Check sheet for the modelled part. Datum: model origin and axes. Units: mm. Give positions to 0.01 mm unless a question says otherwise; leave off trailing zeros. Order: outer loops, then holes, each group sorted by start corner. A loop starts at its lowest first (then second) coordinate and runs counter-clockwise, first axis right, second up. Notation, with made-up numbers: (63.25, 25.25) - (85.25, 25.25) arc R7 ccw to (85.25, 33.25) - close; hole circle Ø1 at (18.5, -26.75). An arc over 180 degrees is marked (long way). Answer in a Markdown table with one row per item.
from build123d import *

# Parameters (mm, degrees)
F1_DEPTH = 13.2


with BuildPart() as f1:
    # F0 (on Right) → F1 (new body)
    with BuildSketch(Plane.YZ):
        with BuildLine():
            ThreePointArc((63.824689, 3.356788), (64.089665, -3.514345), (70, 0))
            ThreePointArc((70, 0), (69.14794, 2.467888), (66.954764, 3.884382))
            ThreePointArc((66.954764, 3.884382), (66.679281, 3.932074), (66.403765, 3.97957))
            ThreePointArc((66.403765, 3.97957), (65.061087, 3.888244), (63.824689, 3.356788))
        make_face()
        with BuildLine():
            ThreePointArc((69, 0), (63.87868, -2.12132), (66, 3))
            ThreePointArc((66, 3), (68.12132, 2.12132), (69, 0))
        make_face(mode=Mode.SUBTRACT)
        with BuildLine():
            ThreePointArc((66.403765, 3.97957), (66.679281, 3.932074), (66.954764, 3.884382))
            ThreePointArc((66.954764, 3.884382), (66.68093, 3.941616), (66.403765, 3.97957))
        make_face()
        with BuildLine():
            ThreePointArc((-64.71288, 2.709856), (-0.470808, 8.340736), (63.824689, 3.356788))
            ThreePointArc((63.824689, 3.356788), (65.061087, 3.888244), (66.403765, 3.97957))
            ThreePointArc((66.403765, 3.97957), (-0.23707, 9.650483), (-66.871424, 3.903924))
            Line((-66.871424, 3.903924), (-66.871424, 2.512486))
            Line((-66.871424, 2.512486), (-64.71288, 2.709856))
        make_face()
    extrude(amount=F1_DEPTH)


solid = f1.part
(1) Cross-section at A-A, the plane x = 11.25. Record the cut outline in (y, z), then the cut area to 3 significant figures.
Geometry says:
| item | result |
|---|---|
| outline | (-66.87, 2.51) - (-64.71, 2.71) arc R391.78 cw to (63.82, 3.36) arc R4 ccw (long way) to (66.95, 3.88) arc R4 ccw to (66.4, 3.98) arc R391.78 ccw to (-66.87, 3.9) - close; hole (66, 3) arc R3 ccw (long way) to (69, 0) arc R3 ccw to start |
| area | 194 mm² |
(2) Gauge pin test, flat ends, axial feed: P1, Ø3, axis at x = 9.5, y = 25, coming from the +Z side; P2, Ø5, axis at y = 66, z = 0, coming from the +X side; P3, Ø1.5, axis at x = 3.5, y = -53, coming from the +Z side; P4, Ø5, axis at x = 7.5, z = 4, coming from the +Y side. Record the tip position at first contact, or that the pin passes through.
Geometry says:
| item | result |
|---|---|
| P1 | z = 8.94 |
| P2 | through |
| P3 | z = 6.15 |
| P4 | y = 69.71 |
(3) Thickness scan on L1, parallel to Y at x = 4.5, z = 0; L2, parallel to Z at x = 3.75, y = 66; L3, parallel to Y at x = 0.75, z = 1.25. Record the ranges inside material, lowest first.
Geometry says:
| item | result |
|---|---|
| L1 | 62 to 63, 69 to 70 |
| L2 | -4 to -3, 3 to 4.05 |
| L3 | 62.2 to 63.27, 68.73 to 69.8 |
(4) Mould release check, pull along Y, two halves, no side actions. Record for faces 1 (the flat face through (6.51, -65.81, 2.61)), 2 (the cylindrical face through (6.51, 0.7, 9.65)), 3 (the flat face through (0, 1, 9)): pulls with the +Y half, pulls with the -Y half, needs draft (parallel to the pull), parting line crosses it, or undercut.
Geometry says:
| item | result |
|---|---|
| face 1 | undercut |
| face 2 | parting line crosses it |
| face 3 | needs draft |
(5) Cross-section at B-B, the plane y = 17. Record the cut outline in (x, z).
Geometry says:
| item | result |
|---|---|
| outline | (0, 8.04) - (13.2, 8.04) - (13.2, 9.28) - (0, 9.28) - close |
